Autodesk Inventor part; units mm, degrees
ref_plane "Начальная плоскость" through (0, 0, 0) normal (1, 0, 0) x (0, 1, 0)
ref_plane "XZ Plane" through (0, 0, 0) normal (0, 1, 0) x (-1, 0, 0)
ref_plane "XY Plane" through (0, 0, 0) normal (0, 0, 1) x (1, 0, 0)
sketch "Основной эскиз" plane through (0, 0, 0) normal (0, 0, 1) x (1, 0, 0)
  line L0 (0, 0) -> (120, 0)
  line L1 (10, 20) -> (10, 15)
  line L2 (0, 20) -> (10, 20)
  line L3 (90, 15) -> (90, 10)
  line L4 (10, 15) -> (90, 15)
  line L5 (120, 10) -> (120, 0)
  line L6 (90, 10) -> (120, 10)
  line L7 (0, 0) -> (0, 20)
  dimension "d4" = 40
  dimension "d5" = 30
  dimension "d6" = 20
revolve "Вращение1" add sketch "Основной эскиз" angle 360 about axis through (0, 0, 0) along (1, 0, 0)
chamfer "Фаска1" distance 2 angle 45 1 edges at (120, -10, 0) measured on face at (110, 9.9676, -0.8047)
properties part number "Вал" material "Steel"
Read the model definition and answer for the solid it produces. Units are mm, in the model's axes. A direction names the side the tool comes from. Give positions to 0.01 mm unless a question says otherwise; leave off trailing zeros. Order: outer loops, then holes, each group sorted by start corner. A loop starts at its lowest first (then second) coordinate and runs counter-clockwise, first axis right, second up. Notation, with made-up numbers: (29, 1.5) -> (82, 1.5) arc R14 ccw to (82, 26.5) -> close; hole circle Ø6 at (-14.75, 71.5). An arc over 180 degrees is marked (long way). Write item = value, one per line.
1. A cutting plane is placed at C-C, the plane x = 74. Write down the section's boundary in (y, z), and give its area (3 significant figures).
Numbers:
outline = circle Ø30 at (0, 0)
area = 707 mm²
2. A cutting plane is placed at D-D, the plane y = 12.5. Write down the section's boundary in (x, z), and give its area (3 significant figures).
Numbers:
outline = (0, -15.61) -> (10, -15.61) -> (10, -8.29) -> (90, -8.29) -> (90, 8.29) -> (10, 8.29) -> (10, 15.61) -> (0, 15.61) -> close
area = 1,640 mm²
3. For faces 1 (the face through (0, 0, 0)), 2 (the face through (90, 3, -10)), determine the directions among +Z, -Z, +X, -X, +Y, -Y from which every point of the face is accessible in a straight line to the end or side of a thin tool.
Numbers:
face_1 = +Z, -Z, -X, +Y, -Y
face_2 = +X
4. Straight lines are drawn through the part: line 1 along Z through (x, y) = (102.5, 0.5); line 2 along X through (y, z) = (15.5, -10); line 3 along X through (y, z) = (12.5, 5). For each, find the intervals that lie inside material, in ascending order.
Numbers:
line_1 = -9.99 to 9.99
line_2 = 0 to 10
line_3 = 0 to 90
5. A cutting plane is placed at A-A, the plane z = 0. Write down the section's boundary in (x, y).
Numbers:
outline = (0, -20) -> (10, -20) -> (10, -15) -> (90, -15) -> (90, -10) -> (118, -10) -> (120, -8) -> (120, 8) -> (118, 10) -> (90, 10) -> (90, 15) -> (10, 15) -> (10, 20) -> (0, 20) -> close
6. Given pin 1 (2 mm diameter, centred on y = 5.5, z = 16, fed in from +X); pin 2 (6 mm diameter, centred on x = 15, y = -3.5, fed in from +Z); pin 3 (10 mm diameter, centred on x = 64, y = -1.5, fed in from -Z), each flat-ended and moving along its own axis, determine where each tip first touches the part or whether it passes through.
Numbers:
pin_1 = 10
pin_2 = 14.99
pin_3 = -15
